Geometry check sheet. Reference: the model listing, model coordinates, mm. A direction names the side the tool comes from. Round coordinates to 2 decimals unless told otherwise and drop trailing zeros. Loops run counter-clockwise (first coordinate to the right, second up) from the corner with the lowest first, then second, coordinate; pieces in that order, holes last. Notation, with made-up numbers: (-14.75, 39) -> (22.25, 39) arc R23 ccw to (22.25, 50) -> close; hole circle Ø8 at (39, 27.5). An arc over 180 degrees is marked (long way). Use a Markdown table: item, result. Add a question column.
Q1. Gauge pin test, flat ends, axial feed: P1, Ø5, axis at y = 4.5, z = -3.5, coming from the -X side; P2, Ø5, axis at x = 786.5, y = 16, coming from the -Z side; P3, Ø8, axis at y = 6.5, z = 2.5, coming from the +X side; P4, Ø12.5, axis at x = 48.5, y = 11.5, coming from the +Z side. Record the tip position at first contact, or that the pin passes through.
Q2. Set-up check for faces 1 (the face through (46, 12, -9.5)), 2 (the face through (746, 25, 0)), 3 (the face through (44, 12, 9.5)): record each of +Z, -Z, +X, -X, +Y, -Y from which the full face is reachable in a straight line by a thin tool's end or side.
Q3. Sectioned sample at A-A, the plane z = 1. Enter the section's corners in (x, y).
Q4. Material ranges on L1, parallel to Y at x = 440, z = -20; L2, parallel to X at y = 4.25, z = -3.5; L3, parallel to X at y = 6.25, z = 18.5, recorded low to high.
```python
from build123d import *

# Parameters (mm, degrees)
EXTRUDE_1_DEPTH               = 25
CUT_EXTRUDE_START             = -6
CUT_EXTRUDE_1_DEPTH           = 6
PATTERN_LINEAR_1_COUNT        = 2
PATTERN_LINEAR_1_PITCH        = 300
PATTERN_START                 = -6
PATTERN_LINEAR_3_COPY_1_DEPTH = 6
PATTERN_LINEAR_3_COPY_2_DEPTH = 6
MIRROR_START                  = -6
MIRROR_5_COPY_1_DEPTH         = 6
MIRROR_5_COPY_2_DEPTH         = 6
MIRROR_5_COPY_3_DEPTH         = 6
MIRROR_5_COPY_4_DEPTH         = 6
MIRROR_5_COPY_5_DEPTH         = 6
CUT_EXTRUDE_3_DEPTH           = 6
CUT_EXTRUDE_4_DEPTH           = 6


with BuildPart() as part:
    # 草图1 → 凸台-拉伸1 (new body)
    with BuildSketch(Plane(origin=(0, 0, 0), x_dir=(1, 0, 0), z_dir=(0, 1, 0))):
        Polygon((0, 0), (0, -9.5), (90, -9.5), (90, -24), (1513, -24), (1465, 24), (90, 24), (90, 9.5), (0, 9.5), align=None)
    extrude(amount=EXTRUDE_1_DEPTH)

    # 草图2 → 切除-拉伸1 (cut)
    with BuildSketch(Plane(origin=(0, 25, 0), x_dir=(1, 0, 0), z_dir=(0, 1, 0)).offset(CUT_EXTRUDE_START)):
        Polygon((112.5, 24), (120, 16.5), (160, 16.5), (167.5, 24), align=None)
    cut_extrude_1 = extrude(amount=-CUT_EXTRUDE_1_DEPTH, mode=Mode.SUBTRACT)

    # 阵列(线性)1: 切除-拉伸1 ×2
    with Locations(*[(i * PATTERN_LINEAR_1_PITCH, 0, 0) for i in range(1, PATTERN_LINEAR_1_COUNT)]):
        add(cut_extrude_1, mode=Mode.SUBTRACT)

    # 阵列(线性)3 copy 1 sketch → 阵列(线性)3 copy 1 (cut)
    with BuildSketch(Plane(origin=(650, 25, 0), x_dir=(1, 0, 0), z_dir=(0, 1, 0)).offset(PATTERN_START)):
        Polygon((112.5, 24), (120, 16.5), (160, 16.5), (167.5, 24), align=None)
    extrude(amount=-PATTERN_LINEAR_3_COPY_1_DEPTH, mode=Mode.SUBTRACT)

    # 阵列(线性)3 copy 2 sketch → 阵列(线性)3 copy 2 (cut)
    with BuildSketch(Plane(origin=(1000, 25, 0), x_dir=(1, 0, 0), z_dir=(0, 1, 0)).offset(PATTERN_START)):
        Polygon((112.5, 24), (120, 16.5), (160, 16.5), (167.5, 24), align=None)
    extrude(amount=-PATTERN_LINEAR_3_COPY_2_DEPTH, mode=Mode.SUBTRACT)

    # 镜向3: 切除-拉伸1 across plane
    add(cut_extrude_1.mirror(Plane.XY), mode=Mode.SUBTRACT)

    # 镜向5 copy 1 sketch → 镜向5 copy 1 (cut)
    with BuildSketch(Plane(origin=(300, 25, 0), x_dir=(1, 0, 0), z_dir=(0, 1, 0)).offset(MIRROR_START)):
        Polygon((112.5, -24), (120, -16.5), (160, -16.5), (167.5, -24), align=None)
    extrude(amount=-MIRROR_5_COPY_1_DEPTH, mode=Mode.SUBTRACT)

    # 镜向5 copy 2 sketch → 镜向5 copy 2 (cut)
    with BuildSketch(Plane(origin=(0, 25, 0), x_dir=(1, 0, 0), z_dir=(0, 1, 0)).offset(MIRROR_START)):
        Polygon((112.5, -24), (120, -16.5), (160, -16.5), (167.5, -24), align=None)
    extrude(amount=-MIRROR_5_COPY_2_DEPTH, mode=Mode.SUBTRACT)

    # 镜向5 copy 3 sketch → 镜向5 copy 3 (cut)
    with BuildSketch(Plane(origin=(650, 25, 0), x_dir=(1, 0, 0), z_dir=(0, 1, 0)).offset(MIRROR_START)):
        Polygon((112.5, -24), (120, -16.5), (160, -16.5), (167.5, -24), align=None)
    extrude(amount=-MIRROR_5_COPY_3_DEPTH, mode=Mode.SUBTRACT)

    # 镜向5 copy 4 sketch → 镜向5 copy 4 (cut)
    with BuildSketch(Plane(origin=(1000, 25, 0), x_dir=(1, 0, 0), z_dir=(0, 1, 0)).offset(MIRROR_START)):
        Polygon((112.5, -24), (120, -16.5), (160, -16.5), (167.5, -24), align=None)
    extrude(amount=-MIRROR_5_COPY_4_DEPTH, mode=Mode.SUBTRACT)

    # 镜向5 copy 5 sketch → 镜向5 copy 5 (cut)
    with BuildSketch(Plane(origin=(0, 25, 0), x_dir=(1, 0, 0), z_dir=(0, 1, 0)).offset(MIRROR_START)):
        Polygon((112.5, -24), (120, -16.5), (160, -16.5), (167.5, -24), align=None)
    extrude(amount=-MIRROR_5_COPY_5_DEPTH, mode=Mode.SUBTRACT)

    # 草图3 → 切除-拉伸3 (cut)
    with BuildSketch(Plane(origin=(0, 25, 0), x_dir=(1, 0, 0), z_dir=(0, 1, 0)).offset(CUT_EXTRUDE_START)):
        Polygon((1430.5, 24), (1438, 16.5), (1472.5, 16.5), (1465, 24), align=None)
    extrude(amount=-CUT_EXTRUDE_3_DEPTH, mode=Mode.SUBTRACT)

    # 草图4 → 切除-拉伸4 (cut)
    with BuildSketch(Plane(origin=(0, 25, 0), x_dir=(1, 0, 0), z_dir=(0, 1, 0)).offset(CUT_EXTRUDE_START)):
        Polygon((1430.5, -24), (1438, -16.5), (1505.5, -16.5), (1513, -24), align=None)
    extrude(amount=-CUT_EXTRUDE_4_DEPTH, mode=Mode.SUBTRACT)


solid = part.part
```
Values:
| question | item | result |
|---|---|---|
| 1 | P1 | x = 0 |
| 1 | P2 | z = -16.5 |
| 1 | P3 | x = 1495.5 |
| 1 | P4 | z = 9.5 |
| 2 | face 1 | -Z, -X, +Y, -Y |
| 2 | face 2 | +Z, -Z, +X, -X, +Y |
| 2 | face 3 | +Z, -X, +Y, -Y |
| 3 | outline | (0, 0) -> (1490, 0) -> (1490, 25) -> (0, 25) -> close |
| 4 | L1 | 0 to 13, 19 to 25 |
| 4 | L2 | 0 to 1485.5 |
| 4 | L3 | 90 to 1507.5 |
